For this review, take the finished solid that the model builds, in its own axes (mm). Round coordinates to 2 decimals unless told otherwise and drop trailing zeros. Write each loop counter-clockwise with the first axis right and the second up, starting at its lowest first coordinate (ties: lowest second). Pieces come first, ordered by that corner, then holes. Notation, with made-up numbers: M 52,-16 L 82,-16 A10 ccw 82,0 Z; hole C 29,9.5 d2. An arc over 180 degrees is marked long. Answer in a Markdown table with one row per item.
Solid Edge part; units mm, degrees
sketch "Sketch1" plane through (0, 0, 0) normal (0, 0, 1) x (1, 0, 0)
  spline S0 degree 3 poles (-0.2928, 1.9785) (-0.306, 2.1503) (-0.3512, 2.501) (-0.5844, 2.7739) (-0.7056, 2.9158) knots 0 0 0 0 0.479886 1 1 1 1
  arc A0 (-0.7056, 2.9158) -> (-1.143, 2.7737) centre (0, 0) ccw
  spline S1 degree 3 poles (-0.926, 1.7727) (-1.0163, 1.9195) (-1.1859, 2.2298) (-1.1577, 2.5876) (-1.143, 2.7737) knots 0 0 0 0 0.479886 1 1 1 1
  arc A1 (-0.926, 1.7727) -> (-0.2928, 1.9785) centre (0, 0) cw
extrude "Protrusion1" add sketch "Sketch1" along normal blind 3.5
sketch "Sketch2" plane through (0, 0, 0) normal (0, 0, 1) x (1, 0, 0)
  circle A0 centre (0, 0) radius 1.5
  circle A1 centre (0, 0) radius 2
extrude "Rad" add sketch "Sketch2" along normal blind 3.5
pattern_circular "Pattern1" count 10 over 360 about axis through (0, 0, 0) along (0, 0, 1) of "Protrusion1"
Q1. Insertion check: P1, Ø1, axis at y = 2, z = 1.5, coming from the +X side. The pin has a flat end and moves straight along its axis. Give the tip position at first contact, or say it passes through.
Found:
| item | result |
|---|---|
| P1 | x = 2.56 |
Q2. Take a section at B-B (y = 0). State the section outline as (x, z) points.
Found:
| item | result |
|---|---|
| outline | M -3,0 L -1.5,0 L -1.5,3.5 L -3,3.5 Z; M 1.5,0 L 3,0 L 3,3.5 L 1.5,3.5 Z |
Q3. Take a section at A-A (x = 0). State the section outline as (y, z) points, then the cut area to 3 significant figures.
Found:
| item | result |
|---|---|
| outline | M -2,0 L -1.5,0 L -1.5,3.5 L -2,3.5 Z; M 1.5,0 L 2,0 L 2,3.5 L 1.5,3.5 Z |
| area | 3.50 mm² |
Q4. Mouldability with a two-part tool opening along X and no side actions: class faces 1 (the face through (-2, 0, 0)), 2 (the face through (-1.5, -0.07, 1.73)) as +X half, -X half, draft (parallel to the pull), parting line (faces both ways), or undercut.
Found:
| item | result |
|---|---|
| face 1 | draft |
| face 2 | undercut |
Q5. For probe 1 along Y at (x, z) = (0, 0.9); probe 2 along X at (y, z) = (1.55, 1.35); probe 3 along X at (y, z) = (-1.1, 1.8), list the stretches that pass through material, from the lowest coordinate up.
Found:
| item | result |
|---|---|
| probe 1 | -2 to -1.5, 1.5 to 2 |
| probe 2 | -2.54 to -1.51, -1.26 to 1.26, 1.51 to 2.54 |
| probe 3 | -2.18 to -1.02, 1.02 to 2.18 |
Q6. Take a section at C-C (x = -1). State how many separate pieces and enclosed holes the cut face has, then the cut area to 3 significant figures.
Found:
| item | result |
|---|---|
| separate pieces | 4 |
| enclosed holes | 0 |
| area | 10.8 mm² |
